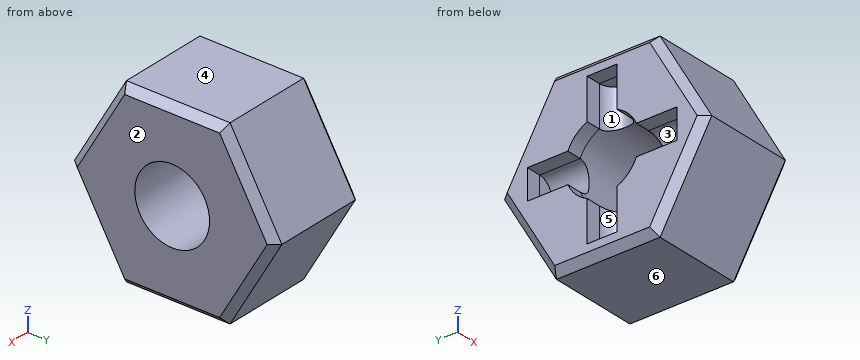
```python
from build123d import *

# Parameters (mm, degrees)
F0_R     = 2.5
F3_DEPTH = 6
F1_R     = 1
F4_DEPTH = 5
F5_DEPTH = 5
F2_R     = 1
F6_DEPTH = 5
F7_DEPTH = 5
F8_SIZE  = 0.5
F9_DEPTH = 1
F10_SIZE = 0.5


with BuildPart() as f3:
    # F0 (on Right) → F3 (new body)
    with BuildSketch(Plane.YZ):
        Polygon((3.4641016151, 6), (-3.4641016151, 6), (-6.9282032303, 0), (-3.4641016151, -6), (3.4641016151, -6), (6.9282032303, 0), align=None)
        Circle(F0_R, mode=Mode.SUBTRACT)
    extrude(amount=F3_DEPTH)

    # F1 (on Front) → F4 (cut)
    with BuildSketch(Plane.XZ):
        Circle(F1_R)
    extrude(amount=-F4_DEPTH, mode=Mode.SUBTRACT)

    # F1 (on Front) → F5 (cut)
    with BuildSketch(Plane.XZ):
        Circle(F1_R)
    extrude(amount=F5_DEPTH, mode=Mode.SUBTRACT)

    # F2 (on Top) → F6 (cut)
    with BuildSketch(Plane.XY):
        Circle(F2_R)
    extrude(amount=-F6_DEPTH, mode=Mode.SUBTRACT)

    # F2 (on Top) → F7 (cut)
    with BuildSketch(Plane.XY):
        Circle(F2_R)
    extrude(amount=F7_DEPTH, mode=Mode.SUBTRACT)

    # F8
    f8_edges = [f3.edges().sort_by_distance(p)[0] for p in [
        (6, 0, -6),
        (6, 5.196152, -3),
        (6, 5.196152, 3),
        (6, 0, 6),
        (6, -5.196152, 3),
        (6, -5.196152, -3),
    ]]
    chamfer(f8_edges, length=F8_SIZE)

    # F9 (add): a face of the model
    f9_faces = [f3.faces().sort_by_distance(p)[0] for p in [
        (0, 5.037407344, 2.9083484861),
    ]]
    extrude(f9_faces, amount=F9_DEPTH)

    # F10
    f10_edges = [f3.edges().sort_by_distance(p)[0] for p in [
        (-1, -5.196152, -3),
        (-1, 5.196152, -3),
        (-1, 0, -6),
        (-1, 0, 6),
        (-1, 5.196152, 3),
        (-1, -5.196152, 3),
    ]]
    chamfer(f10_edges, length=F10_SIZE)


solid = f3.part
```
CAD build for the part. Positions are in the model's coordinates, mm. Face numbers are marked on the shaded views. A direction names the side the tool comes from. Round coordinates to 2 decimals unless told otherwise and drop trailing zeros. Order: outer loops, then holes, each group sorted by start corner. A loop starts at its lowest first (then second) coordinate and runs counter-clockwise, first axis right, second up. Notation, with made-up numbers: (-35, 60) - (-11, 60) arc R4 ccw to (-11, 67) - close; hole circle Ø8 at (10, -5). An arc over 180 degrees is marked (long way). Answer as CSV lines item,"result". Start each with the question number.
1. Pull direction Z, two halves, no side cores. Call the marked faces 3, 4, 5 and 6: +Z half, -Z half, draft (parallel to the pull), parting line (faces both ways), or undercut.
2. Pin check, flat tips, straight feed: pin 1 (0.5 mm diameter, centred on x = -0.5, z = 0.5, fed in from -Y); pin 2 (0.5 mm diameter, centred on x = -0.5, y = -4, fed in from +Z); pin 3 (4 mm diameter, centred on x = 5, z = -3.5, fed in from -Y). Stop position of each tip, or through.
3. Saw through at B-B, the plane z = 2. Write the cut outline in (x, y), and give its area (3 significant figures).
4. Saw through at A-A, the plane y = 0. Write the cut outline in (x, z).
5. Saw through at D-D, the plane y = 2.75. Write the cut outline in (x, z), and give its area (3 significant figures).
6. Tool access for the marked faces 1 and 2: list every direction of +Z, -Z, +X, -X, +Y, -Y with a clear straight run to the whole face (end or side of a thin tool).
7. Drill centre lines: L1, parallel to Z at x = 5.25, y = 1; L2, parallel to Z at x = 2.5, y = 0; L3, parallel to Y at x = 2.5, z = 1. Where is each one in solid material? Low to high. Write a range as [from, to].
8. Saw through at C-C, the plane x = 4.5. Write the cut outline in (y, z), and give its area (3 significant figures).
Model answer:
1,face 3,"undercut"
1,face 4,"+Z half"
1,face 5,"undercut"
1,face 6,"-Z half"
2,pin 1,"stops at y = -6.78"
2,pin 2,"stops at z = 5.5"
2,pin 3,"stops at y = -6.06"
3,outline,"(-1, -5.2) - (-0.5, -5.77) - (5.5, -5.77) - (6, -5.2) - (6, -1.5) - (-1, -1.5) - close; (-1, 1.5) - (6, 1.5) - (6, 5.2) - (5.5, 5.77) - (-0.5, 5.77) - (-1, 5.2) - close"
3,area,"59.3 mm²"
4,outline,"(-1, -5.5) - (-0.5, -6) - (5.5, -6) - (6, -5.5) - (6, -2.5) - (1, -2.5) - (1, -5) - (-1, -5) - close; (-1, 5) - (1, 5) - (1, 2.5) - (6, 2.5) - (6, 5.5) - (5.5, 6) - (-0.5, 6) - (-1, 5.5) - close"
5,outline,"(-1, -5.5) - (-0.5, -6) - (5.5, -6) - (6, -5.5) - (6, 5.5) - (5.5, 6) - (-0.5, 6) - (-1, 5.5) - (-1, 1) - (0, 1) arc R1 cw to (0, -1) - (-1, -1) - close"
5,area,"79.9 mm²"
6,face 1,"-X"
6,face 2,"+Z, -Z, +X, +Y, -Y"
7,L1,"z = [-6, -2.29], [2.29, 6]"
7,L2,"z = [-6, -2.5], [2.5, 6]"
7,L3,"y = [-6.35, -2.29], [2.29, 6.35]"
8,outline,"(-6.93, 0) - (-3.46, -6) - (3.46, -6) - (6.93, 0) - (3.46, 6) - (-3.46, 6) - close; hole circle Ø5 at (0, 0)"
8,area,"105 mm²"
